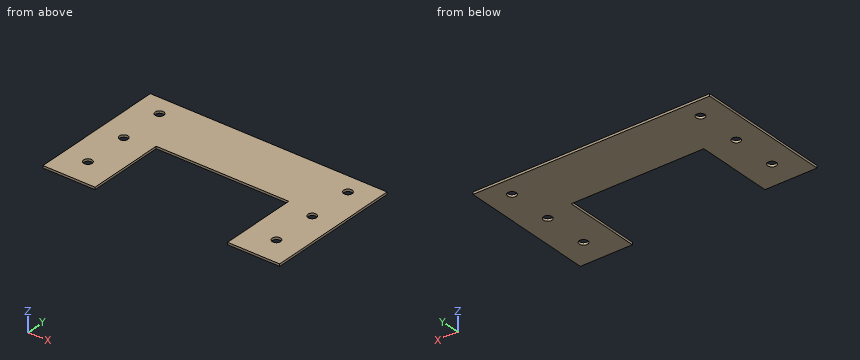
```python
from build123d import *

# Parameters (mm, degrees)
SKETCH_1_R             = 2.25
SM_BASE_FLANGE_1_DEPTH = 1.2


# Sheet-metal steps are written as plain solids
with BuildPart() as part:
    # Sketch 1 → Базовая кромка1 (new body)
    with BuildSketch(Plane.XY):
        Polygon((97.5, 0), (125, 0), (125, 72), (0, 72), (0, 0), (27.5, 0), (27.5, 41), (97.5, 41), align=None)
        with Locations((112.2683, 62)):
            Circle(SKETCH_1_R, mode=Mode.SUBTRACT)
        with Locations((112.2683, 38)):
            Circle(SKETCH_1_R, mode=Mode.SUBTRACT)
        with Locations((112.2683, 14)):
            Circle(SKETCH_1_R, mode=Mode.SUBTRACT)
        with Locations((12.7317, 62)):
            Circle(SKETCH_1_R, mode=Mode.SUBTRACT)
        with Locations((12.7317, 38)):
            Circle(SKETCH_1_R, mode=Mode.SUBTRACT)
        with Locations((12.7317, 14)):
            Circle(SKETCH_1_R, mode=Mode.SUBTRACT)
    extrude(amount=-SM_BASE_FLANGE_1_DEPTH)


solid = part.part
```
Here's how the part is built. I have some questions about the finished solid (model axes, mm). Give positions to 0.01 mm unless a question says otherwise; leave off trailing zeros. Loops run counter-clockwise (first coordinate to the right, second up) from the corner with the lowest first, then second, coordinate; pieces in that order, holes last. Notation, with made-up numbers: (55.5, 30) -> (93.5, 30) arc R29 ccw to (93.5, 64) -> close; hole circle Ø8 at (43, 82). An arc over 180 degrees is marked (long way). Use one line per item in the form item = value. Start each with the question number.
1) Imagine slicing it at C-C (z = -0.85). Please give me the cut outline in (x, y), then the cut area to 3 significant figures.
2) Imagine slicing it at A-A (y = 62). Please give me the cut outline in (x, z).
3) Imagine slicing it at D-D (y = 26). Please give me the cut outline in (x, z).
4) Please list where these lines run through material, in increasing order: line 1 along X through (y, z) = (25, -0.8); line 2 along Y through (x, z) = (70.5, -0.1); line 3 along Y through (x, z) = (14.5, -0.9).
5) Imagine slicing it at B-B (y = 14). Please give me the cut outline in (x, z), then the cut area to 3 significant figures.
6) For P1, Ø0.6, axis at x = 61, z = -0.5, coming from the -Y side, with a flat end and sliding along its axis, tell me the tip position at first contact or that it passes through.
Check values:
q1.outline = (0, 0) -> (27.5, 0) -> (27.5, 41) -> (97.5, 41) -> (97.5, 0) -> (125, 0) -> (125, 72) -> (0, 72) -> close; hole circle Ø4.5 at (12.73, 14); hole circle Ø4.5 at (12.73, 38); hole circle Ø4.5 at (12.73, 62); hole circle Ø4.5 at (112.27, 14); hole circle Ø4.5 at (112.27, 38); hole circle Ø4.5 at (112.27, 62)
q1.area = 6,030 mm^2
q2.outline = (0, -1.2) -> (10.48, -1.2) -> (10.48, 0) -> (0, 0) -> close; (14.98, -1.2) -> (110.02, -1.2) -> (110.02, 0) -> (14.98, 0) -> close; (114.52, -1.2) -> (125, -1.2) -> (125, 0) -> (114.52, 0) -> close
q3.outline = (0, -1.2) -> (27.5, -1.2) -> (27.5, 0) -> (0, 0) -> close; (97.5, -1.2) -> (125, -1.2) -> (125, 0) -> (97.5, 0) -> close
q4.line_1 = 0 to 27.5, 97.5 to 125
q4.line_2 = 41 to 72
q4.line_3 = 0 to 12.61, 15.39 to 36.61, 39.39 to 60.61, 63.39 to 72
q5.outline = (0, -1.2) -> (10.48, -1.2) -> (10.48, 0) -> (0, 0) -> close; (14.98, -1.2) -> (27.5, -1.2) -> (27.5, 0) -> (14.98, 0) -> close; (97.5, -1.2) -> (110.02, -1.2) -> (110.02, 0) -> (97.5, 0) -> close; (114.52, -1.2) -> (125, -1.2) -> (125, 0) -> (114.52, 0) -> close
q5.area = 55.2 mm^2
q6.P1 = 41
